Check sheet for the modelled part. Datum: model origin and axes. Units: mm. A direction names the side the tool comes from. Coordinates: 2 decimals unless noted, no trailing zeros. Write each loop counter-clockwise with the first axis right and the second up, starting at its lowest first coordinate (ties: lowest second). Pieces come first, ordered by that corner, then holes. Notation, with made-up numbers: (-33.75, -38) -> (-17.75, -38) arc R27 cw to (-17.75, -17) -> close; hole circle Ø9 at (-19, 8). An arc over 180 degrees is marked (long way). Put each result on its own line as item: value.
```python
from build123d import *

# Parameters (mm, degrees)
SKETCH005_W     = 12.9
SKETCH005_H     = 11.9
PAD003_DEPTH    = 0.3
FILLET003_R     = 1
PAD004_DEPTH    = 5.55
PAD005_DEPTH    = 0.3
FILLET004_R     = 0.3
SKETCH008_R     = 2.9
PAD006_DEPTH    = 9
SKETCH009_R     = 1.95
POCKET002_DEPTH = 5
CHAMFER_SIZE    = 0.5
SKETCH010_W     = 0.5
SKETCH010_H     = 0.8
POCKET003_DEPTH = 9


with BuildPart() as part:
    # Sketch005 → Pad003 (new body)
    with BuildSketch(Plane.XY):
        Rectangle(SKETCH005_W, SKETCH005_H)
    extrude(amount=-PAD003_DEPTH)

    # Fillet003
    fillet003_edges = [part.edges().sort_by_distance(p)[0] for p in [
        (-6.45, -5.95, -0.15),
        (-6.45, 5.95, -0.15),
        (6.45, 5.95, -0.15),
        (6.45, -5.95, -0.15),
    ]]
    fillet(fillet003_edges, radius=FILLET003_R)

    # Sketch006 (on Face2 of Fillet003) → Pad004 (join)
    with BuildSketch(Plane.XY):
        Polygon((-4.901521, 6.25), (4.898479, 6.25), (4.898479, 5.95), (-4.9, 5.95), align=None)
        Polygon((4.901521, -6.25), (-4.9, -6.25), (-4.9, -5.949996), (4.9, -5.949996), align=None)
    extrude(amount=-PAD004_DEPTH)

    # Sketch007 (on Face21 of Pad004) → Pad005 (join)
    with BuildSketch(Plane(origin=(0, 0, -5.55), x_dir=(1, 0, 0), z_dir=(0, 0, -1))):
        with BuildLine():
            ThreePointArc((-3.05, 5.95), (-2.3, 5.2), (-1.55, 5.95))
            Line((-1.55, 5.95), (-1.55, 6.25))
            Line((-3.05, 6.25), (-1.55, 6.25))
            Line((-3.05, 6.25), (-3.05, 5.95))
        make_face()
        with BuildLine():
            ThreePointArc((1.55, 5.95), (2.3, 5.2), (3.05, 5.95))
            Line((3.05, 5.95), (3.05, 6.25))
            Line((1.55, 6.25), (3.05, 6.25))
            Line((1.55, 6.25), (1.55, 5.95))
        make_face()
        with BuildLine():
            ThreePointArc((-1.55, -5.95), (-2.3, -5.2), (-3.05, -5.95))
            Line((-3.05, -5.95), (-3.05, -6.25))
            Line((-3.05, -6.25), (-1.55, -6.25))
            Line((-1.55, -6.25), (-1.55, -5.95))
        make_face()
        with BuildLine():
            ThreePointArc((3.05, -5.95), (2.3, -5.2), (1.55, -5.95))
            Line((1.55, -5.95), (1.55, -6.25))
            Line((1.55, -6.25), (3.05, -6.25))
            Line((3.05, -6.25), (3.05, -5.95))
        make_face()
    extrude(amount=PAD005_DEPTH)

    # Fillet004
    fillet004_edges = [part.edges().sort_by_distance(p)[0] for p in [
        (2.3, -6.25, -5.85),
        (-2.3, -6.25, -5.85),
        (2.3, 6.25, -5.85),
        (-2.3, 6.25, -5.85),
        (-0.001521, 6.25, 0),
        (0.000761, -6.25, 0),
    ]]
    fillet(fillet004_edges, radius=FILLET004_R)

    # Sketch008 (on Face1 of Fillet004) → Pad006 (join)
    with BuildSketch(Plane.XY):
        Circle(SKETCH008_R)
    extrude(amount=PAD006_DEPTH)

    # Sketch009 (on Face22 of Pad006) → Pocket002 (cut)
    with BuildSketch(Plane.XY.offset(9)):
        Circle(SKETCH009_R)
    extrude(amount=-POCKET002_DEPTH, mode=Mode.SUBTRACT)

    # Chamfer
    chamfer_edges = [part.edges().sort_by_distance(p)[0] for p in [
        (-2.9, 0, 9),
    ]]
    chamfer(chamfer_edges, length=CHAMFER_SIZE)

    # Sketch010 (on Face4 of Chamfer) → Pocket003 (cut)
    with BuildSketch(Plane.XY.offset(9)):
        with Locations((2.7, 0)):
            Rectangle(SKETCH010_W, SKETCH010_H)
    extrude(amount=-POCKET003_DEPTH, mode=Mode.SUBTRACT)


solid = part.part
```
Q1. Cross-section at A-A (z = -1.25). Record the cut outline in (x, y), plus the area to 3 significant figures.
Recorded:
outline: (-4.9, -6.25) -> (4.9, -6.25) -> (4.9, -5.95) -> (-4.9, -5.95) -> close; (-4.9, 5.95) -> (4.9, 5.95) -> (4.9, 6.25) -> (-4.9, 6.25) -> close
area: 5.88 mm2
Q2. Cross-section at D-D (z = 5). Record the cut outline in (x, y).
Recorded:
outline: (2.45, -0.4) -> (2.45, 0.4) -> (2.87, 0.4) arc R2.9 ccw (long way) to (2.87, -0.4) -> close; hole circle Ø3.9 at (0, 0)
Q3. Material ranges on line 1 along Y through (x, z) = (-4.75, -3); line 2 along Y through (x, z) = (0, 4.5); line 3 along Z through (x, y) = (-2.5, 5.5), recorded low to high.
Recorded:
line 1: y = -6.25 to -5.95, 5.95 to 6.25
line 2: y = -2.9 to -1.95, 1.95 to 2.9
line 3: z = -5.85 to -5.55, -0.3 to 0
Q4. Tool access check on faces 5 (the flat face through (-1, 2, 9)), 6 (the flat face through (0, 0, 4)), 7 (the flat face through (0, 5.95, -3)). Record the directions out of +Z, -Z, +X, -X, +Y, -Y that give a thin tool (end or side, any length) a straight path to the whole face; none if there is none.
Recorded:
face 5: +Z, +X, -X, +Y, -Y
face 6: +Z
face 7: +X, -X
Q5. Cross-section at B-B (x = -4.25). Record the cut outline in (y, z).
Recorded:
outline: (-6.25, -5.55) -> (-5.95, -5.55) -> (-5.95, -0.3) -> (5.95, -0.3) -> (5.95, -5.55) -> (6.25, -5.55) -> (6.25, -0.3) arc R0.3 ccw to (5.95, 0) -> (-5.95, 0) arc R0.3 ccw to (-6.25, -0.3) -> close
Q6. Mould release check, pull along Y, two halves, no side actions. Record for faces 1 (the flat face through (0, -6.25, -3)), 2 (the flat face through (2.45, 0, 5)), 3 (the cylindrical face through (-2.9, 0.1, 4.2)), 4 (the flat face through (0, 6.25, -3)): released by +Y, released by -Y, zero draft, split by the parting line, or undercut.
Recorded:
face 1: released by -Y
face 2: undercut
face 3: split by the parting line
face 4: released by +Y
Q7. Depth check by flat-ended pin: P1, Ø1.2, axis at x = -1, y = 0.5, coming from the +Z side; P2, Ø0.8, axis at x = -2, y = 5.5, coming from the +Z side; P3, Ø0.5, axis at x = 2.5, z = 4, coming from the +Y side; P4, Ø1.5, axis at y = 4.5, z = 4, coming from the +X side. Enter the tip coordinate at first touch or a pass-through.
Recorded:
P1: stops at z = 4
P2: stops at z = 0
P3: stops at y = 1.83
P4: passes through
Q8. Cross-section at C-C (y = 0). Record the cut outline in (x, z).
Recorded:
outline: (-6.45, -0.3) -> (6.45, -0.3) -> (6.45, 0) -> (2.45, 0) -> (2.45, 8.95) -> (2.4, 9) -> (1.95, 9) -> (1.95, 4) -> (-1.95, 4) -> (-1.95, 9) -> (-2.4, 9) -> (-2.9, 8.5) -> (-2.9, 0) -> (-6.45, 0) -> close
